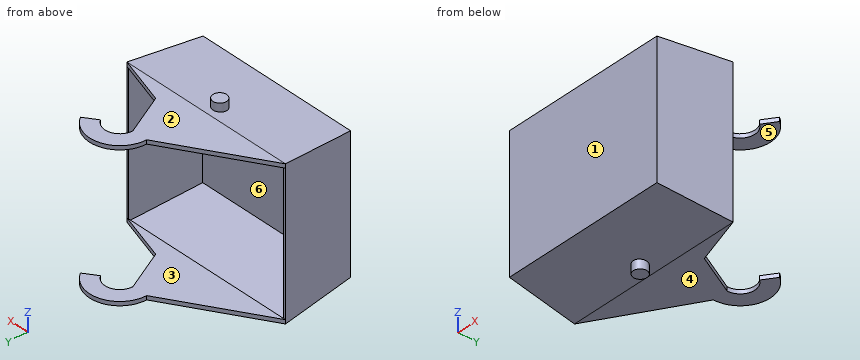
```python
from build123d import *

# Parameters (mm, degrees)
SKETCH1_W           = 266.7
SKETCH1_H           = 215.9
SKETCH1_W_2         = 260.35
SKETCH1_H_2         = 209.55
BOSS_EXTRUDE1_DEPTH = 114.3
BOSS_EXTRUDE1_TAPER = -5
SKETCH1_5_W         = 260.35
SKETCH1_5_H         = 209.55
BOSS_EXTRUDE2_DEPTH = 3.175
BOSS_EXTRUDE2_TAPER = -5
SKETCH3_W           = 280.349908482
SKETCH3_H           = 229.549908482
SKETCH3_W_2         = 240.350091518
SKETCH3_H_2         = 189.550091518
CUT_EXTRUDE1_DEPTH  = 111.125
CUT_EXTRUDE1_TAPER  = 5
BOSS_EXTRUDE3_START = -114.774954
BOSS_EXTRUDE3_DEPTH = 3.175
BOSS_EXTRUDE4_START = -114.774954
SKETCH7_R           = 11
BOSS_EXTRUDE4_DEPTH = 15


with BuildPart() as part:
    # Sketch1 → Boss-Extrude1 (new body)
    with BuildSketch(Plane(origin=(0, 0, 0), x_dir=(1, 0, 0), z_dir=(0, 1, 0))):
        Rectangle(SKETCH1_W, SKETCH1_H)
        Rectangle(SKETCH1_W_2, SKETCH1_H_2, mode=Mode.SUBTRACT)
    extrude(amount=BOSS_EXTRUDE1_DEPTH, taper=BOSS_EXTRUDE1_TAPER)

    # Sketch1<5> → Boss-Extrude2 (add)
    with BuildSketch(Plane(origin=(0, 0, 0), x_dir=(1, 0, 0), z_dir=(0, 1, 0))):
        Rectangle(SKETCH1_5_W, SKETCH1_5_H)
    extrude(amount=BOSS_EXTRUDE2_DEPTH, taper=BOSS_EXTRUDE2_TAPER)

    # Sketch3 → Cut-Extrude1 (cut)
    with BuildSketch(Plane(origin=(0, 114.3, 0), x_dir=(1, 0, 0), z_dir=(0, 1, 0))):
        Rectangle(SKETCH3_W, SKETCH3_H)
        Rectangle(SKETCH3_W_2, SKETCH3_H_2, mode=Mode.SUBTRACT)
    extrude(amount=-CUT_EXTRUDE1_DEPTH, taper=CUT_EXTRUDE1_TAPER, mode=Mode.SUBTRACT)

    # Sketch5 → Boss-Extrude3 (add, symmetric)
    with BuildSketch(Plane.XY.offset(BOSS_EXTRUDE3_START)):
        with BuildLine():
            Line((-143.349954241, 114.3), (5.849954241, 205.3))
            ThreePointArc((5.849954241, 205.3), (39.905581805, 251.746015501), (94.442658798, 233.23317245))
            Line((94.442658798, 233.23317245), (73.963857691, 218.893761542))
            ThreePointArc((73.963857691, 218.893761542), (47.423226793, 227.903091733), (30.849954241, 205.3))
            Line((30.849954241, 205.3), (63.349954241, 139.3))
            Line((63.349954241, 139.3), (143.349954241, 114.3))
            Line((143.349954241, 114.3), (-143.349954241, 114.3))
        make_face()
    boss_extrude3 = extrude(amount=BOSS_EXTRUDE3_DEPTH, both=True)

    # Sketch7 → Boss-Extrude4 (add)
    with BuildSketch(Plane.XY.offset(BOSS_EXTRUDE4_START)):
        with Locations((0, 92.3)):
            Circle(SKETCH7_R)
    boss_extrude4 = extrude(amount=-BOSS_EXTRUDE4_DEPTH)

    # Mirror5: Boss-Extrude3, Boss-Extrude4 across plane
    add(boss_extrude3.mirror(Plane.XY))
    add(boss_extrude4.mirror(Plane.XY))


solid = part.part
```
Source: CAD feature listing. Evaluate the final solid. Frame: model axes, mm. Face numbers are marked on the shaded views. A direction names the side the tool comes from. Round coordinates to 2 decimals unless told otherwise and drop trailing zeros. Loops run counter-clockwise (first coordinate to the right, second up) from the corner with the lowest first, then second, coordinate; pieces in that order, holes last. Notation, with made-up numbers: (-29.75, -24.75) - (-8.75, -24.75) arc R18 cw to (-8.75, -8.75) - close; hole circle Ø6 at (38, 76). An arc over 180 degrees is marked (long way). Use CSV: the item, a comma, the result in double quotes.
Q1. Pin query (flat end, axial travel): pin 1 Ø6 at (y, z) = (85.5, -17) entering from -X; pin 2 Ø10 at (x, y) = (83.5, 57.5) entering from -Z; pin 3 Ø10 at (x, y) = (-64.5, 132) entering from +Z. Return the tip coordinate at first contact, or that it passes through.
Reported:
pin 1,"x = -141.09"
pin 2,"z = -113.42"
pin 3,"z = 117.95"
Q2. Ray query, line 1 along Z through (x, y) = (-4, 184.5); line 2 along Y through (x, z) = (5, -103.5) (3 decimals); line 3 along X through (y, z) = (42.5, 53). Return the intervals inside material, ascending.
Reported:
line 1,"-117.95 to -111.6, 111.6 to 117.95"
line 2,"0 to 3.175"
line 3,"-137.07 to -133.89, 133.89 to 137.07"
Q3. Reachability of the marked faces 4, 5 and 6 from +Z, -Z, +X, -X, +Y, -Y: full face, straight path, thin tool, end or side. Return the list, or none.
Reported:
face 4,"-Z, +X, -X, +Y"
face 5,"+X, -X, +Y"
face 6,"+Y"
Q4. Mould query, pull axis Z, two halves, no side actions, for the marked faces 1, 2 and 3. Classes: pulls with the +Z half, pulls with the -Z half, needs draft (parallel to the pull), parting line crosses it, or undercut.
Reported:
face 1,"needs draft"
face 2,"pulls with the +Z half"
face 3,"undercut"
Q5. Section query A-A, the plane y = 213. Output: boundary loops of the cut face in (x, z).
Reported:
outline,"(6.46, -117.95) - (32.14, -117.95) - (32.14, -111.6) - (6.46, -111.6) - close; (6.46, 111.6) - (32.14, 111.6) - (32.14, 117.95) - (6.46, 117.95) - close"
